Here's how the part is built. I have some questions about the finished solid (model axes, mm). Face numbers are marked on the shaded views. A direction names the side the tool comes from. Coordinates: 2 decimals unless noted, no trailing zeros. Order: outer loops, then holes, each group sorted by start corner. A loop starts at its lowest first (then second) coordinate and runs counter-clockwise, first axis right, second up. Notation, with made-up numbers: M 89.5,48 L 135.5,48 A24 cw 135.5,73 Z; hole C -30.5,58 d10. An arc over 180 degrees is marked long. Answer as CSV lines item,"result". Start each with the question number.
```python
from build123d import *

# Parameters (mm, degrees)
SKETCH_W        = 40
SKETCH_H        = 20
SKETCH_R        = 1.85
PAD_DEPTH       = 8.5
POCKET001_DEPTH = 1
SKETCH003_R     = 2.4
POCKET_DEPTH    = 8.501
SKETCH004_W     = 11
SKETCH004_H     = 1
POCKET002_DEPTH = 20.001
FILLET_R        = 6


with BuildPart() as part:
    # Sketch → Pad (new body)
    with BuildSketch(Plane.XY):
        Rectangle(SKETCH_W, SKETCH_H)
        with Locations((-15, 6.5)):
            Circle(SKETCH_R, mode=Mode.SUBTRACT)
        with Locations((15, 6.5)):
            Circle(SKETCH_R, mode=Mode.SUBTRACT)
        with Locations((15, -6.5)):
            Circle(SKETCH_R, mode=Mode.SUBTRACT)
        with Locations((-15, -6.5)):
            Circle(SKETCH_R, mode=Mode.SUBTRACT)
    extrude(amount=PAD_DEPTH)

    # Sketch002 → Pocket001 (cut)
    with BuildSketch(Plane(origin=(0, 0, 0), x_dir=(1, 0, 0), z_dir=(0, 0, -1))):
        Polygon((20, 13.717063), (10.020782, 11.721405), (10.020782, 2.538416), (20, 2.538416), align=None)
        Polygon((10.020782, -2.538416), (20, -2.538416), (20, -12.706139), (10.020782, -11.721405), align=None)
    pocket001 = extrude(amount=-POCKET001_DEPTH, mode=Mode.SUBTRACT)

    # Mirrored: Pocket001 across Sketch002 V_Axis
    add(pocket001.mirror(Plane(origin=(0, 0, 0), x_dir=(0, 0, -1), z_dir=(1, 0, 0))), mode=Mode.SUBTRACT)

    # Sketch003 (on DatumPlane) → Pocket (cut, through all)
    with BuildSketch(Plane(origin=(0, 0, 0), x_dir=(1, 0, 0), z_dir=(0, 0, -1))):
        with Locations((0, 5.73236)):
            Circle(SKETCH003_R)
        with Locations((0, -5.73236)):
            Circle(SKETCH003_R)
    extrude(amount=-POCKET_DEPTH, mode=Mode.SUBTRACT)

    # Sketch004 (on DatumPlane) → Pocket002 (cut, through all)
    with BuildSketch(Plane(origin=(0, 10, 0), x_dir=(-1, 0, 0), z_dir=(0, 1, 0))):
        with Locations((0, 8.5)):
            Rectangle(SKETCH004_W, SKETCH004_H)
    extrude(amount=-POCKET002_DEPTH, mode=Mode.SUBTRACT)

    # Fillet
    fillet_edges = [part.edges().sort_by_distance(p)[0] for p in [
        (-10.020782, 2.538416, 0.5),
        (-10.020782, -2.538416, 0.5),
        (10.020782, -2.538416, 0.5),
        (10.020782, 2.538416, 0.5),
        (20, 10, 4.75),
        (20, -10, 4.75),
        (-20, -10, 4.75),
        (-20, 10, 4.75),
    ]]
    fillet(fillet_edges, radius=FILLET_R)


solid = part.part
```
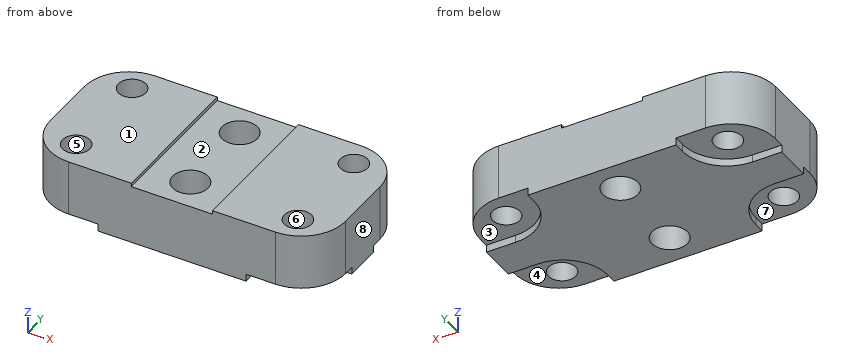
1) Suppose I cut it at D-D on y = 5.25. Please give me the cut outline in (x, z).
2) I need wall thicknesses on line 1 (Y direction, x = 0, z = 4.25); line 2 (Y direction, x = -15, z = 6.5); line 3 (X direction, y = 6, z = 4.75). Which ranges of each line are inside material? Lowest first, please. Write a range as [from, to].
3) Will these pins go through, and if not, where does the flat tip stop? pin 1 Ø0.8 at (x, z) = (-18, 0.5) entering from +Y; pin 2 Ø0.6 at (y, z) = (4.5, 8) entering from -X; pin 3 Ø8 at (x, y) = (-15.5, 7) entering from -Z.
4) Suppose I cut it at A-A on x = 0. Please give me the cut outline in (y, z).
5) Suppose I cut it at B-B on y = -1. Please give me the cut outline in (x, z).
6) Which directions (+Z, -Z, +X, -X, +Y, -Y) give clear straight access to the entire face, cutting with the end or side of a thin tool? Please do the marked faces 1, 2, 3 and 4.
7) Suppose I cut it at C-C on z = 5. Please give me the cut outline in (x, y).
8) If we mould it in two halves opening along X, with no side actions, what happens to the marked faces 5, 6, 7 and 8? For each: released by +X, released by -X, zero draft, split by the parting line, or undercut.
Output:
1,outline,"M -19.87,1 L -16.36,1 L -16.36,8.5 L -19.87,8.5 Z; M -13.64,1 L -11,1 L -11,0 L -2.35,0 L -2.35,8 L -5.5,8 L -5.5,8.5 L -13.64,8.5 Z; M 2.35,0 L 11,0 L 11,1 L 13.64,1 L 13.64,8.5 L 5.5,8.5 L 5.5,8 L 2.35,8 Z; M 16.36,1 L 19.87,1 L 19.87,8.5 L 16.36,8.5 Z"
2,line 1,"[-10, -8.13], [-3.33, 3.33], [8.13, 10]"
2,line 2,"[-9.92, -8.35], [-4.65, 4.65], [8.35, 9.92]"
2,line 3,"[-19.66, -16.78], [-13.22, -2.39], [2.39, 13.22], [16.78, 19.66]"
3,pin 1,"y = 2.54"
3,pin 2,"x = -20"
3,pin 3,"z = 1"
4,outline,"M -10,0 L -8.13,0 L -8.13,8 L -10,8 Z; M -3.33,0 L 3.33,0 L 3.33,8 L -3.33,8 Z; M 8.13,0 L 10,0 L 10,8 L 8.13,8 Z"
5,outline,"M -20,0 L 20,0 L 20,8.5 L 5.5,8.5 L 5.5,8 L -5.5,8 L -5.5,8.5 L -20,8.5 Z"
6,face 1,"+Z, +X, -X, +Y, -Y"
6,face 2,"+Z, +Y, -Y"
6,face 3,"-Z, +X, +Y"
6,face 4,"-Z, +X, -Y"
7,outline,"M -20,-4 A6 ccw -14,-10 L 14,-10 A6 ccw 20,-4 L 20,4 A6 ccw 14,10 L -14,10 A6 ccw -20,4 Z; hole C -15,-6.5 d3.7; hole C -15,6.5 d3.7; hole C 0,-5.73 d4.8; hole C 0,5.73 d4.8; hole C 15,-6.5 d3.7; hole C 15,6.5 d3.7"
8,face 5,"undercut"
8,face 6,"undercut"
8,face 7,"zero draft"
8,face 8,"released by +X"
